Could you check a few things on this drawing? It's one solid part, dimensions in mm from its lowest x, y, z. A direction names the side the tool comes from. Coordinates: 2 decimals unless noted, no trailing zeros. Write each loop counter-clockwise with the first axis right and the second up, starting at its lowest first coordinate (ties: lowest second). Pieces come first, ordered by that corner, then holes. Notation, with made-up numbers: (-0.5, 30) - (20.5, 30) arc R12 cw to (20.5, 51) - close; hole circle Ø4 at (87, -32). An arc over 180 degrees is marked (long way). Write item = value, one per line. Start each with the question number.
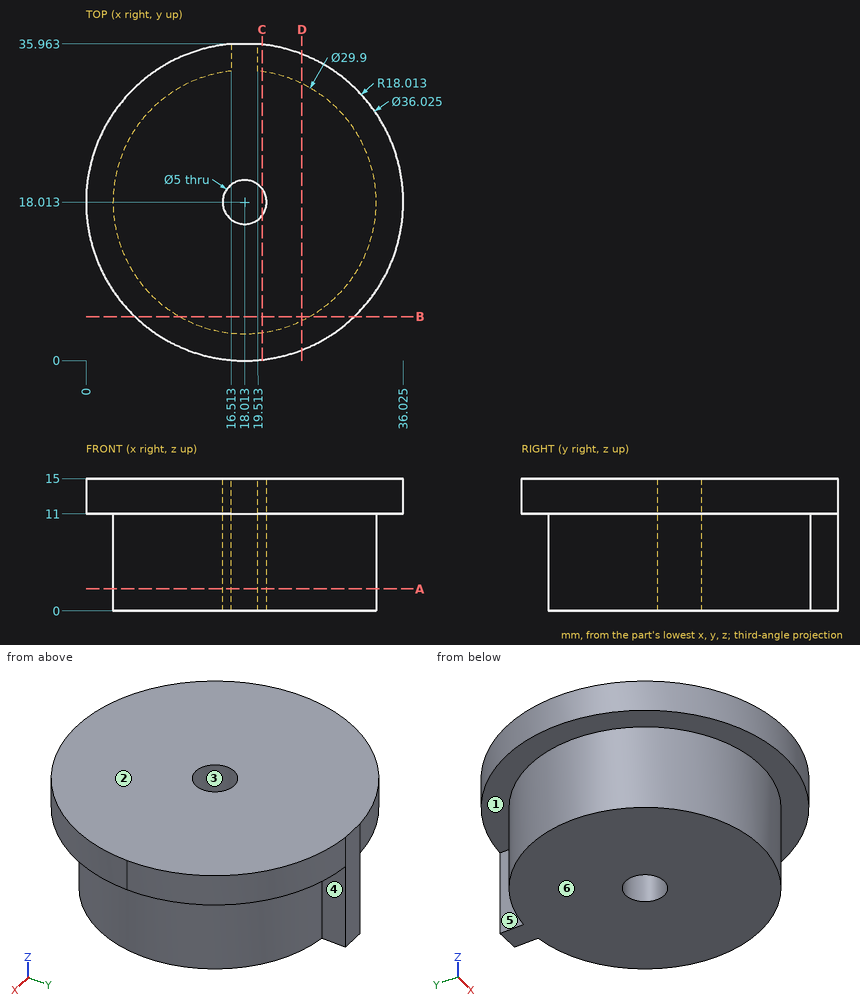
1) If I drill on probe 1 along Z at (x, y) = (33, 9.5); probe 2 along X at (y, z) = (17, 12) (1 decimal); probe 3 along X at (y, z) = (17, 4.75), over which ranges is the centre line in solid material (lowest first)? Write a range as [from, to].
2) Which directions (+Z, -Z, +X, -X, +Y, -Y) give clear straight access to the entire face, cutting with the end or side of a thin tool? Please do the marked faces 1 and 2.
3) For P1, Ø1.5, axis at y = 12.5, z = 5.5, coming from the +X side; P2, Ø0.9, axis at y = 34.5, z = 8, coming from the +X side; P3, Ø4, axis at x = 20.5, z = 12.5, coming from the -Y side, each with a flat end and sliding along its axis, tell me the tip position at first contact or that it passes through.
4) Suppose I cut it at B-B on y = 5. Please give me the cut outline in (x, z).
5) Suppose I cut it at A-A on z = 2.5. Please give me the cut outline in (x, y).
6) Suppose I cut it at C-C on x = 20. Please give me the cut outline in (y, z) (1 decimal), plus the area to 3 significant figures.
7) Thinking about a two-plate mould opening in X: for the marked faces 3, 4, 5 and 6, which applies, +X half, -X half, draft (parallel to the pull), parting line (faces both ways), or undercut?
8) Suppose I cut it at D-D on x = 24.5. Please give me the cut outline in (y, z).
Reply:
q1.probe_1 = [11, 15]
q1.probe_2 = [0, 15.7], [20.3, 36]
q1.probe_3 = [3.1, 15.73], [20.3, 32.93]
q2.face_1 = -Z
q2.face_2 = +Z, +X, -X, +Y, -Y
q3.P1 = 32.18
q3.P2 = 19.51
q3.P3 = 0.01
q4.outline = (5.56, 11) - (10.65, 11) - (10.65, 0) - (25.37, 0) - (25.37, 11) - (30.47, 11) - (30.47, 15) - (5.56, 15) - close
q5.outline = (16.51, 32.89) arc R14.95 ccw (long way) to (19.51, 32.89) - (19.51, 35.96) - (16.51, 35.96) - close; hole circle Ø5 at (18.01, 18.01)
q6.outline = (0.1, 11) - (3.2, 11) - (3.2, 0) - (16.5, 0) - (16.5, 15) - (0.1, 15) - close; (19.5, 0) - (32.8, 0) - (32.8, 11) - (35.9, 11) - (35.9, 15) - (19.5, 15) - close
q6.area = 424 mm^2
q7.face_3 = undercut
q7.face_4 = +X half
q7.face_5 = -X half
q7.face_6 = draft
q8.outline = (1.21, 11) - (4.54, 11) - (4.54, 0) - (31.48, 0) - (31.48, 11) - (34.82, 11) - (34.82, 15) - (1.21, 15) - close
